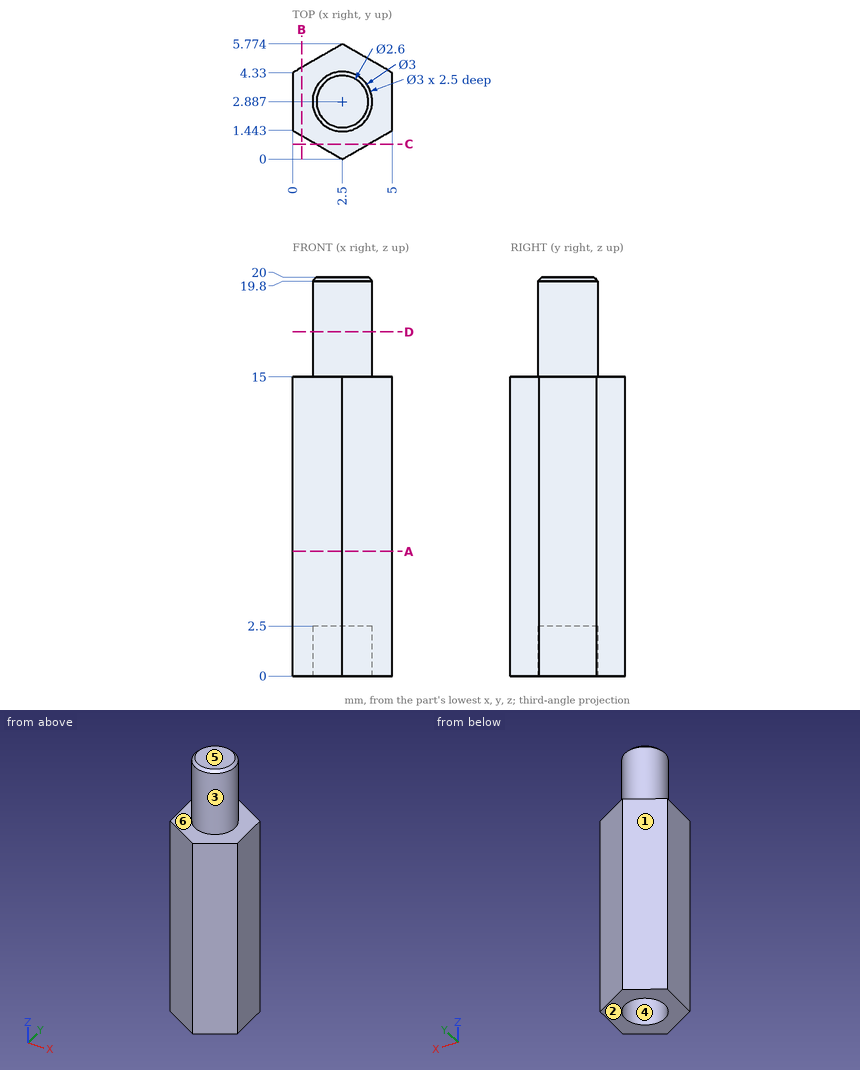
Print and shaded views of the part. All mm, measured from the part's lowest x, y and z. A direction names the side the tool comes from. Round coordinates to 2 decimals unless told otherwise and drop trailing zeros. Order: outer loops, then holes, each group sorted by start corner. A loop starts at its lowest first (then second) coordinate and runs counter-clockwise, first axis right, second up.
Q1. Slice it at C-C (y = 0.75). Write the cut outline in (x, z).
Q2. Which spindle directions (+Z, -Z, +X, -X, +Y, -Y) get a long thin tool onto all of the face, cutting with end or side? Do the marked faces 5 and 6. Say none if no direction does.
Q3. Two-plate mould, pull along Y, no slides. Class the marked faces 1, 2, 3 and 4: pulls with the +Y half, pulls with the -Y half, needs draft (parallel to the pull), parting line crosses it, or undercut.
Q4. Slice it at D-D (z = 17.25). Write the cut outline in (x, y).
Q5. Wall check: L1, parallel to Z at x = 2, y = 0.5; L2, parallel to Z at x = 1.75, y = 3.6; L3, parallel to Y at x = 2.65, z = 8.5 (1 decimal). Give the ranges that are in metal, low to high.
Q6. Slice it at A-A (z = 6.25). Write the cut outline in (x, y).
Q7. Slice it at B-B (x = 0.45). Write the cut outline in (y, z), and give its area (3 significant figures).
Results below:
1. outline: (1.2, 0) - (3.8, 0) - (3.8, 15) - (1.2, 15) - close
2. face 5: +Z, +X, -X, +Y, -Y
2. face 6: +Z
3. face 1: pulls with the +Y half
3. face 2: needs draft
3. face 3: parting line crosses it
3. face 4: undercut
4. outline: circle Ø3 at (2.5, 2.89)
5. L1: z = 0 to 15
5. L2: z = 2.5 to 20
5. L3: y = 0.1 to 5.7
6. outline: (0, 1.44) - (2.5, 0) - (5, 1.44) - (5, 4.33) - (2.5, 5.77) - (0, 4.33) - close
7. outline: (1.18, 0) - (4.59, 0) - (4.59, 15) - (1.18, 15) - close
7. area: 51.1 mm2
